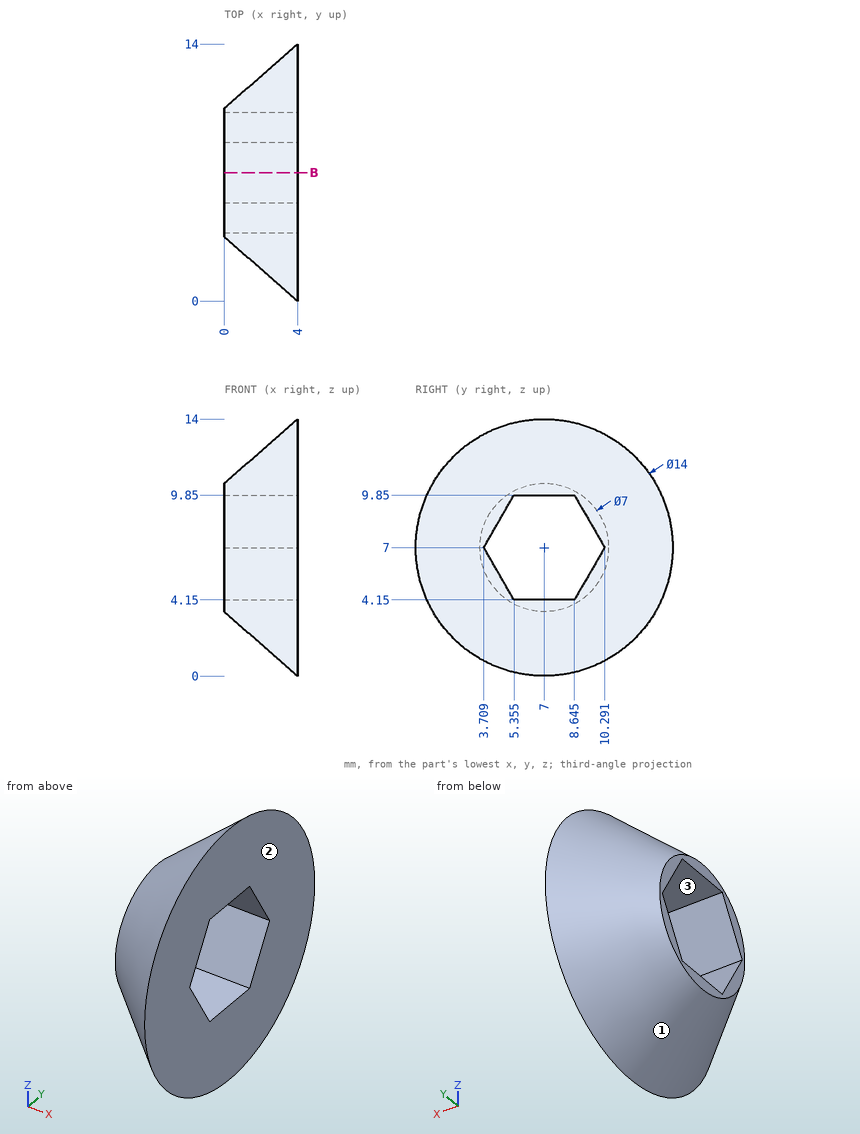
For this review, use the dimensioned drawing (mm, ordinates from the lowest corner) and the shaded views. Give positions to 0.01 mm unless a question says otherwise; leave off trailing zeros. Write each loop counter-clockwise with the first axis right and the second up, starting at its lowest first coordinate (ties: lowest second). Pieces come first, ordered by that corner, then holes. Notation, with made-up numbers: M -28,-3.5 L -4,-3.5 A26 cw -4,20.5 Z; hole C 57,2.25 d5. An arc over 180 degrees is marked long. Answer as a JSON object with one key per item and string values. Group by question number.
Item 1: Consider section B-B on y = 7. Write out the cut boundary in (x, z).
Item 2: For probe 1 along Z at (x, y) = (2.5, 10) (1 decimal); probe 2 along Z at (x, y) = (3.7, 10) (1 decimal); probe 3 along Y at (x, z) = (1.15, 5.75), list the stretches that pass through material, from the lowest coordinate up. Write a range as [from, to].
Item 3: For pin 1 Ø1.5 at (x, y) = (2, 10.5) entering from -Z; pin 2 Ø1 at (x, y) = (1.5, 6.5) entering from +Z; pin 3 Ø1.5 at (x, y) = (1, 8.5) entering from +Z (1 decimal), all flat-tipped, find the tip position at first contact; note any pin that passes through.
Item 4: Draft analysis for pull direction Y (two halves, no side actions). For the marked faces 1, 2 and 3, state which applies: +Y half, -Y half, draft (parallel to the pull), parting line (faces both ways), or undercut.
Check result:
{
 "1": {"outline": "M 0,3.5 L 4,0 L 4,4.15 L 0,4.15 Z; M 0,9.85 L 4,9.85 L 4,14 L 0,10.5 Z"},
 "2": {"probe 1": "z = [2.2, 6.5], [7.5, 11.8]", "probe 2": "z = [1, 6.5], [7.5, 13]", "probe 3": "y = [2.67, 4.43], [9.57, 11.33]"},
 "3": {"pin 1": "stops at z = 2.09", "pin 2": "stops at z = 12.23", "pin 3": "stops at z = 11.8"},
 "4": {"face 1": "parting line", "face 2": "draft", "face 3": "undercut"}
}
